Read the model definition and answer for the solid it produces. Units are mm, in the model's axes. A direction names the side the tool comes from. Give positions to 0.01 mm unless a question says otherwise; leave off trailing zeros. Write each loop counter-clockwise with the first axis right and the second up, starting at its lowest first coordinate (ties: lowest second). Pieces come first, ordered by that corner, then holes. Notation, with made-up numbers: (-29.5, 9) -> (-17.5, 9) arc R21 ccw to (-17.5, 25) -> close; hole circle Ø4 at (58.5, -40). An arc over 180 degrees is marked (long way). Write item = value, one per line.
from build123d import *

# Parameters (mm, degrees)
SKETCH_1_W          = 84
SKETCH_1_H          = 31.8
EXTRUDE_1_DEPTH     = 6
SKETCH_2_W          = 80
SKETCH_2_H          = 3
CUT_EXTRUDE_1_DEPTH = 3
EXTRUDE_2_DEPTH     = 5
SKETCH_4_R          = 5
SKETCH_4_R_2        = 6
CUT_EXTRUDE_2_DEPTH = 91.488894346
SKETCH_3_3_W        = 22
SKETCH_3_3_H        = 3.2
SKETCH_3_3_H_2      = 6.8
CUT_EXTRUDE_3_DEPTH = 91.0179982


with BuildPart() as part:
    # Sketch 1 → Extrude 1 (new body)
    with BuildSketch(Plane(origin=(0, 0, 0), x_dir=(1, 0, 0), z_dir=(0, 1, 0))):
        with Locations((42, -15.9)):
            Rectangle(SKETCH_1_W, SKETCH_1_H)
    extrude(amount=EXTRUDE_1_DEPTH)

    # Sketch 2 → Cut-Extrude 1 (cut)
    with BuildSketch(Plane(origin=(0, 6, 0), x_dir=(1, 0, 0), z_dir=(0, 1, 0))):
        with Locations((42, -27.8)):
            Rectangle(SKETCH_2_W, SKETCH_2_H)
    extrude(amount=-CUT_EXTRUDE_1_DEPTH, mode=Mode.SUBTRACT)

    # Sketch 3 → Extrude 2 (add)
    with BuildSketch(Plane(origin=(0, 6, 0), x_dir=(1, 0, 0), z_dir=(0, 1, 0))):
        Polygon((31, 0), (0, 0), (0, -26.3), (5.8, -26.3), (5.8, -3.2), (31, -3.2), align=None)
        Polygon((84, 0), (53, 0), (53, -3.2), (78.2, -3.2), (78.2, -26.3), (84, -26.3), align=None)
    extrude(amount=EXTRUDE_2_DEPTH)

    # Sketch 4 → Cut-Extrude 2 (cut, through all)
    with BuildSketch(Plane(origin=(0, 0, 0), x_dir=(-1, 0, 0), z_dir=(0, 0, -1))):
        with Locations((-63.35, 12.3)):
            Circle(SKETCH_4_R)
        with Locations((-18.25, 14)):
            Circle(SKETCH_4_R_2)
    extrude(amount=-CUT_EXTRUDE_2_DEPTH, mode=Mode.SUBTRACT)

    # Sketch 3_3 → Cut-Extrude 3 (cut, through all)
    with BuildSketch(Plane(origin=(0, 6, 0), x_dir=(1, 0, 0), z_dir=(0, 1, 0))):
        with Locations((42, -1.6)):
            Rectangle(SKETCH_3_3_W, SKETCH_3_3_H)
        with Locations((42, -6.6)):
            Rectangle(SKETCH_3_3_W, SKETCH_3_3_H_2)
    extrude(amount=-CUT_EXTRUDE_3_DEPTH, mode=Mode.SUBTRACT)


solid = part.part
(1) Given P1, Ø7, axis at x = 25, z = 11, coming from the +Y side; P2, Ø1.5, axis at x = 21, y = 7.5, coming from the +Z side; P3, Ø4, axis at x = 45.5, y = 2.5, coming from the -Z side, each flat-ended and moving along its own axis, determine where each tip first touches the part or whether it passes through.
Checks:
P1 = 6
P2 = 3.2
P3 = 10
(2) Consider L1, parallel to X at y = 7, z = 23.5; L2, parallel to X at y = 3.25, z = 8.5; L3, parallel to Z at x = 17, y = 5.25. Determine where each line is inside the solid, lowest interval first.
Checks:
L1 = 0 to 5.8, 78.2 to 84
L2 = 0 to 31, 53 to 84
L3 = 0 to 26.3, 29.3 to 31.8
(3) The part is cut by section A-A on y = 5.25. Determine the outline of the cut face in (x, z).
Checks:
outline = (0, 0) -> (31, 0) -> (31, 10) -> (53, 10) -> (53, 0) -> (84, 0) -> (84, 31.8) -> (0, 31.8) -> close; hole (2, 26.3) -> (82, 26.3) -> (82, 29.3) -> (2, 29.3) -> close
(4) For a pull along X with two mould halves and no side action, classify faces 1 (the flat face through (41, 0, 16)), 2 (the flat face through (65, 7, 3.2)), 3 (the flat face through (0, 5, 16)) as released by +X, released by -X, zero draft, split by the parting line, or undercut.
Checks:
face_1 = zero draft
face_2 = undercut
face_3 = released by -X
(5) The part is cut by section B-B on x = 56. Determine the outline of the cut face in (y, z).
Checks:
outline = (0, 0) -> (11, 0) -> (11, 3.2) -> (6, 3.2) -> (6, 26.3) -> (3, 26.3) -> (3, 29.3) -> (6, 29.3) -> (6, 31.8) -> (0, 31.8) -> close
(6) The part is cut by section C-C on z = 17. Determine the outline of the cut face in (x, y).
Checks:
outline = (0, 0) -> (84, 0) -> (84, 11) -> (78.2, 11) -> (78.2, 6) -> (5.8, 6) -> (5.8, 11) -> (0, 11) -> close
(7) A tool of negligible diameter and unlimited length cuts with its end or side. For faces 4 (the flat face through (41, 3, 28)), 5 (the flat face through (18, 7, 3.2)), 6 (the flat face through (53, 4, 4)), from which of +Z, -Z, +X, -X, +Y, -Y can it reach the whole face along a straight path? Write none if from no direction.
Checks:
face_4 = +Y
face_5 = +Z, +Y
face_6 = -Z, +Y, -Y
(8) The part is cut by section D-D on y = 2. Determine the outline of the cut face in (x, z).
Checks:
outline = (0, 0) -> (31, 0) -> (31, 10) -> (53, 10) -> (53, 0) -> (84, 0) -> (84, 31.8) -> (0, 31.8) -> close
